Input: part model. Units: mm. Frame: model coordinates. Face numbers are marked on the shaded views. A direction names the side the tool comes from. Give positions to 0.01 mm unless a question says otherwise; leave off trailing zeros. Order: outer loops, then holes, each group sorted by start corner. A loop starts at its lowest first (then second) coordinate and runs counter-clockwise, first axis right, second up. Notation, with made-up numbers: (-6.75, -13) - (42.25, -13) arc R23 cw to (42.25, 3) - close; hole circle Ø10 at (8.25, 85.5). An arc over 180 degrees is marked (long way). Answer in a Markdown table with one row per item. Add a question column.
1. Section query B-B on y = 0.5. Return loops of the section in (x, z).
2. Mould query, pull axis Y, two halves, no side actions, for the marked faces 4, 5, 6 and 7. Classes: released by +Y, released by -Y, zero draft, split by the parting line, or undercut.
3. Contact query for flat-ended pins moving along their axis: pin 1 (2 mm diameter, centred on x = -11, z = -3.5, fed in from +Y); pin 2 (2.5 mm diameter, centred on y = 0, z = -3, fed in from +X); pin 3 (5 mm diameter, centred on y = -14.5, z = -5, fed in from -X). Output: stop coordinate, or through.
4. Section query C-C on x = -28. Return loops of the section in (y, z), and give its area (3 significant figures).
5. Access query for the marked faces 1, 2 and 3. Directions: +Z, -Z, +X, -X, +Y, -Y. A direction counts if a zero-diameter tool reaches every point of the face in a straight line with its end or side. Return the directions, or none.
6. Ray query, line 1 (Y direction, x = -19.5, z = -7.5); line 2 (X direction, y = -16.25, z = -1.75); line 3 (X direction, y = -7, z = -2.75). Return the intervals inside material, ascending. Write a range as [from, to].
Autodesk Inventor part; units mm, degrees
ref_plane "Work Plane2" through (-20.3233, -0.3, -20.2296) normal (0, 1, 0) x (0, 0, 1)
ref_plane "YZ Plane" through (0, 0, 0) normal (1, 0, 0) x (0, 1, 0)
ref_plane "XZ Plane" through (0, 0, 0) normal (0, 1, 0) x (-1, 0, 0)
sketch "Sketch1" plane through (0, 0, 0) normal (0, 0, 1) x (1, 0, 0)
  arc A0 (-31.9035, -17) -> (-29.9035, -19) centre (-29.9035, -17) ccw
  line L0 (-29.9035, -19) -> (-2, -19)
  arc A1 (-2, -19) -> (0, -17) centre (-2, -17) ccw
  line L1 (0, 1) -> (0, -17)
  arc A2 (0, 1) -> (-2, 3) centre (-2, 1) ccw
  line L2 (-2, 3) -> (-29.9035, 3)
  arc A3 (-29.9035, 3) -> (-31.9035, 1) centre (-29.9035, 1) ccw
  line L3 (-31.9035, -17) -> (-31.9035, 1)
  line L4 (-17.2029, -18.3) -> (-17.2029, -16)
  line L5 (-28.9035, -16) -> (-17.2029, -16)
  line L6 (-28.9035, 0) -> (-28.9035, -16)
  line L7 (-17.2029, 0) -> (-28.9035, 0)
  line L8 (-17.2029, 0) -> (-17.2029, 2.3)
  line L9 (-17.2029, 2.3) -> (-14.6938, 2.3)
  line L10 (-14.6938, 2.3) -> (-14.6938, 0)
  line L11 (-3, 0) -> (-14.6938, 0)
  line L12 (-3, 0) -> (-3, -16)
  line L13 (-14.6938, -16) -> (-3, -16)
  line L14 (-14.6938, -16) -> (-14.6938, -18.3)
  line L15 (-17.2029, -18.3) -> (-14.6938, -18.3)
  line L16 (-14.6938, -16) -> (-17.2029, -16)
  line L17 (-14.6938, 0) -> (-17.2029, 0)
  line L18 (-16.9029, -16) -> (-14.9938, -16)
  line L19 (-14.9938, -16) -> (-14.9938, -18)
  line L20 (-14.9938, -18) -> (-16.9029, -18)
  line L21 (-16.9029, -18) -> (-16.9029, -16)
  line L22 (-16.9029, 2) -> (-14.9938, 2)
  line L23 (-14.9938, 2) -> (-14.9938, 0)
  line L24 (-14.9938, 0) -> (-16.9029, 0)
  line L25 (-16.9029, 0) -> (-16.9029, 2)
  point P0 (0, 0)
  dimension "d5" = 0.3
  dimension "d6" = 0
  dimension "d7" = 0.3
  dimension "d8" = 0.3
  dimension "d9" = 0.3
  dimension "d10" = 0.3
  dimension "d11" = 0.3
  dimension "d12" = 0
extrude "Extrusion1" add sketch "Sketch1" against normal blind 14.9 contours L16 L19 L20 L21 | L25 L22 L23 L17
ref_plane "Work Plane1" through (0, 0, 0) normal (0, 0, 1) x (1, 0, 0)
sketch "Sketch2" plane through (0, 0, 0) normal (0, 0, 1) x (1, 0, 0)
  arc A0 (-31.9035, -17) -> (-29.9035, -19) centre (-29.9035, -17) ccw
  line L0 (-29.9035, -19) -> (-2, -19)
  arc A1 (-2, -19) -> (0, -17) centre (-2, -17) ccw
  line L1 (0, 1) -> (0, -17)
  arc A2 (0, 1) -> (-2, 3) centre (-2, 1) ccw
  line L2 (-2, 3) -> (-29.9035, 3)
  arc A3 (-29.9035, 3) -> (-31.9035, 1) centre (-29.9035, 1) ccw
  line L3 (-31.9035, -17) -> (-31.9035, 1)
  line L4 (-17.2029, -18.3) -> (-17.2029, -16)
  line L5 (-28.9035, -16) -> (-17.2029, -16)
  line L6 (-28.9035, 0) -> (-28.9035, -16)
  line L7 (-17.2029, 0) -> (-28.9035, 0)
  line L8 (-17.2029, 0) -> (-17.2029, 2.3)
  line L9 (-17.2029, 2.3) -> (-14.6938, 2.3)
  line L10 (-14.6938, 2.3) -> (-14.6938, 0)
  line L11 (-3, 0) -> (-14.6938, 0)
  line L12 (-3, 0) -> (-3, -16)
  line L13 (-14.6938, -16) -> (-3, -16)
  line L14 (-14.6938, -16) -> (-14.6938, -18.3)
  line L15 (-17.2029, -18.3) -> (-14.6938, -18.3)
  line L16 (-17.2029, 0) -> (-14.6938, 0)
  line L17 (-14.6938, 0) -> (-14.6938, 2.3)
  line L18 (-14.6938, 2.3) -> (-17.2029, 2.3)
  line L19 (-17.2029, 2.3) -> (-17.2029, 0)
  line L20 (-17.2029, -18.3) -> (-14.6938, -18.3)
  line L21 (-14.6938, -18.3) -> (-14.6938, -16)
  line L22 (-14.6938, -16) -> (-17.2029, -16)
  line L23 (-17.2029, -16) -> (-17.2029, -18.3)
  point P0 (0, 0)
extrude "Extrusion2" add sketch "Sketch2" along normal blind 3 contours L3 A3 L2 A2 L1 A1 L0 A0 | L4 L22 L14 L15 | L5 L6 L7 L16 L11 L12 L13 L22 | L8 L9 L10 L16
fillet "Fillet1" radius 2 8 edges at (-31.3177, -18.4142, 3) (-31.9035, -8, 3) (-31.3177, 2.4142, 3) (-15.9518, 3, 3) (-0.5858, 2.4142, 3) (0, -8, 3) (-0.5858, -18.4142, 3) (-15.9518, -19, 3)
sketch "Sketch3" plane through (0, 0, 0) normal (0, 0, -1) x (-1, 0, 0)
  arc A0 (29.9035, -19) -> (31.9035, -17) centre (29.9035, -17) ccw
  line L0 (29.9035, -19) -> (2, -19)
  arc A1 (0, -17) -> (2, -19) centre (2, -17) ccw
  line L1 (0, 1) -> (0, -17)
  arc A2 (2, 3) -> (0, 1) centre (2, 1) ccw
  line L2 (2, 3) -> (29.9035, 3)
  arc A3 (31.9035, 1) -> (29.9035, 3) centre (29.9035, 1) ccw
  line L3 (31.9035, -17) -> (31.9035, 1)
  line L4 (17.2029, -18.3) -> (17.2029, -16)
  line L5 (28.9035, -16) -> (17.2029, -16)
  line L6 (28.9035, 0) -> (28.9035, -16)
  line L7 (17.2029, 0) -> (28.9035, 0)
  line L8 (17.2029, 0) -> (17.2029, 2.3)
  line L9 (17.2029, 2.3) -> (14.6938, 2.3)
  line L10 (14.6938, 2.3) -> (14.6938, 0)
  line L11 (3, 0) -> (14.6938, 0)
  line L12 (3, 0) -> (3, -16)
  line L13 (14.6938, -16) -> (3, -16)
  line L14 (14.6938, -16) -> (14.6938, -18.3)
  line L15 (17.2029, -18.3) -> (14.6938, -18.3)
  line L16 (14.9938, 0) -> (16.9029, 0)
  line L17 (14.9938, 0) -> (14.9938, -0.3)
  line L18 (14.9938, -0.3) -> (3.3, -0.3)
  line L19 (3.3, -0.3) -> (3.3, -1.8)
  line L20 (3.3, -1.8) -> (28.6035, -1.8)
  line L21 (28.6035, -0.3) -> (16.9029, -0.3)
  line L22 (16.9029, 0) -> (16.9029, -0.3)
  line L23 (28.6035, -1.8) -> (28.6035, -0.3)
  line L24 (3, -8) -> (28.9035, -8) construction
  line L25 (14.9938, -16) -> (16.9029, -16)
  line L26 (14.9938, -16) -> (14.9938, -15.7)
  line L27 (14.9938, -15.7) -> (3.3, -15.7)
  line L28 (3.3, -15.7) -> (3.3, -14.2)
  line L29 (3.3, -14.2) -> (28.6035, -14.2)
  line L30 (28.6035, -15.7) -> (16.9029, -15.7)
  line L31 (16.9029, -16) -> (16.9029, -15.7)
  line L32 (28.6035, -14.2) -> (28.6035, -15.7)
  line L33 (3.3, -1.8) -> (3.3, -14.2)
  line L34 (4.8, -14.2) -> (4.8, -1.8)
  line L35 (28.6035, -1.8) -> (28.6035, -14.2)
  line L36 (27.1035, -14.2) -> (27.1035, -1.8)
  point P0 (0, 0)
  dimension "d13" = 0.3
  dimension "d14" = 0.3
  dimension "d15" = 1.5
  dimension "d16" = 0.3
  dimension "d17" = 0.3
  dimension "d20" = 1.5
  dimension "d21" = 1.5
extrude "Extrusion3" add sketch "Sketch3" along normal blind 3 contours L16 L22 L21 L23 L20 L19 L18 L17 | L20 L34 L29 L33 | L35 L29 L36 L20 | L29 L32 L30 L31 L25 L26 L27 L28
sketch "Sketch4" plane through (-14.9938, -18, -14.9) normal (1, 0, 0) x (0, 0, -1)
  line L0 (-14.9, -0.3) -> (2.2893, -0.3)
  line L1 (-14.9, 2) -> (-14.9, -0.3)
  line L2 (2.2893, 2) -> (-14.9, 2)
  line L3 (2.2893, 2) -> (2.2893, -0.3)
  line L4 (0, 2) -> (0, 0)
  line L5 (-14.9, 0) -> (0, 0)
  line L6 (-14.9, 2.3) -> (-14.9, 0)
  line L7 (-14.9, 2.3) -> (-11.9, 2.3)
  line L8 (-11.9, 2.3) -> (-11.9, 2)
  line L9 (-11.9, 2) -> (0, 2)
  line L10 (0, 18) -> (0, 20)
  line L11 (-14.9, 20) -> (0, 20)
  line L12 (-14.9, 20) -> (-14.9, 17.7)
  line L13 (-14.9, 17.7) -> (-11.9, 17.7)
  line L14 (-11.9, 17.7) -> (-11.9, 18)
  line L15 (-11.9, 18) -> (0, 18)
  line L16 (-7.45, 2) -> (-11.9, 4.6913)
  line L17 (-11.9, 4.6913) -> (-11.9, 2.3)
  line L18 (-11.9, 10) -> (3.9744, 10) construction
  line L19 (-7.45, 18) -> (-11.9, 15.3087)
  line L20 (-11.9, 15.3087) -> (-11.9, 17.7)
  point P0 (-14.9, 18)
extrude "Extrusion4" add sketch "Sketch4" against normal up to surface (1.9092 mm away) contours L8 L17 L16 L2 | L19 L20 L14 L15
sketch "Sketch6" plane through (0, 0, 0) normal (0, 0, -1) x (-1, 0, 0)
  line L0 (27.1035, -1.8) -> (4.8, -1.8)
  line L1 (4.8, -1.8) -> (4.8, -14.2)
  line L2 (4.8, -14.2) -> (27.1035, -14.2)
  line L3 (27.1035, -14.2) -> (27.1035, -1.8)
  line L4 (14.9938, -13.3087) -> (16.9029, -13.3087)
  line L5 (14.9938, -2.6913) -> (16.9029, -2.6913)
  line L6 (14.9938, -2.6913) -> (5.6913, -2.6913)
  line L7 (5.6913, -2.6913) -> (5.6913, -13.3087)
  line L8 (5.6913, -13.3087) -> (14.9938, -13.3087)
  line L9 (16.9029, -13.3087) -> (26.2122, -13.3087)
  line L10 (26.2122, -13.3087) -> (26.2122, -2.6913)
  line L11 (26.2122, -2.6913) -> (16.9029, -2.6913)
  point P0 (0, 0)
  dimension "d24" = 0.8913
  dimension "d25" = 0.8913
  dimension "d26" = 0.8913
extrude "Extrusion5" add sketch "Sketch6" along normal up to surface (3 mm away)
sketch "Sketch7" plane through (0, 0, 0) normal (0, 0, -1) x (-1, 0, 0)
  line L0 (14.9938, -2.6913) -> (14.9938, -0.3)
  line L1 (3.3, -0.3) -> (14.9938, -0.3)
  line L2 (3.3, -15.7) -> (3.3, -0.3)
  line L3 (14.9938, -15.7) -> (3.3, -15.7)
  line L4 (14.9938, -13.3087) -> (14.9938, -15.7)
  line L5 (5.6913, -13.3087) -> (14.9938, -13.3087)
  line L6 (5.6913, -2.6913) -> (5.6913, -13.3087)
  line L7 (14.9938, -2.6913) -> (5.6913, -2.6913)
  line L8 (16.9029, -0.3) -> (16.9029, -2.6913)
  line L9 (26.2122, -2.6913) -> (16.9029, -2.6913)
  line L10 (26.2122, -13.3087) -> (26.2122, -2.6913)
  line L11 (16.9029, -13.3087) -> (26.2122, -13.3087)
  line L12 (16.9029, -13.3087) -> (16.9029, -15.7)
  line L13 (28.6035, -15.7) -> (16.9029, -15.7)
  line L14 (28.6035, -0.3) -> (28.6035, -15.7)
  line L15 (16.9029, -0.3) -> (28.6035, -0.3)
  line L16 (5.6913, -8) -> (10.3425, -13.3087)
  line L17 (5.6913, -8) -> (10.3425, -2.6913)
  line L18 (21.5576, -2.6913) -> (26.2122, -8)
  line L19 (26.2122, -8) -> (21.5576, -13.3087)
  point P0 (0, 0)
extrude "Extrusion6" add sketch "Sketch7" along normal up to surface (3 mm away) contours L17 L6 L7 | L16 L5 L6 | L9 L10 L18 | L10 L11 L19
sketch "Sketch8" plane through (0, 0, -14.9) normal (0, 0, -1) x (-1, 0, 0)
  line L0 (16.9029, 2) -> (16.9029, 0)
  line L1 (14.9938, 0) -> (14.9938, 2)
  line L2 (16.9029, 0) -> (14.9938, 0)
  line L3 (13.4938, 2) -> (18.4028, 2)
  line L4 (18.4028, 2) -> (18.4028, 0)
  line L5 (18.4028, 0) -> (13.4938, 0)
  line L6 (13.4938, 0) -> (13.4938, 2)
  line L7 (3.3, -15.7) -> (3.3, -0.3)
  line L8 (28.6035, -0.3) -> (28.6035, -15.7)
  line L9 (3.3, -8) -> (28.6035, -8) construction
  line L10 (13.4938, -18) -> (18.4028, -18)
  line L11 (18.4028, -18) -> (18.4028, -16)
  line L12 (18.4028, -16) -> (13.4938, -16)
  line L13 (13.4938, -16) -> (13.4938, -18)
  point P0 (0, 0)
  dimension "d31" = 4.909
  dimension "d32" = 1.9092
  dimension "d33" = 1.4999
  dimension "d34" = 0
  dimension "d35" = 2
  dimension "d36" = 2
extrude "Extrusion7" add sketch "Sketch8" against normal up to surface (14.9 mm away)
sketch "Sketch9" plane through (-14.9938, -16, 0) normal (1, 0, 0) x (0, 0, -1)
  line L0 (0, 0) -> (7.45, 0)
  line L1 (7.45, 0) -> (3, 2.6913)
  line L2 (3, 2.6913) -> (3, 0.3)
  line L3 (0, 0.3) -> (3, 0.3)
  line L4 (0, 0) -> (0, 0.3)
  line L5 (7.45, 16) -> (0, 16)
  line L6 (0, 16) -> (0, 15.7)
  line L7 (0, 15.7) -> (3, 15.7)
  line L8 (3, 13.3087) -> (3, 15.7)
  line L9 (3, 13.3087) -> (7.45, 16)
  point P0 (0, 16)
extrude "Extrusion8" add sketch "Sketch9" along normal up to surface (1.4999 mm away)
sketch "Sketch10" plane through (-16.9029, -16, 0) normal (-1, 0, 0) x (0, 0, 1)
  line L0 (-7.45, 0) -> (0, 0)
  line L1 (0, 0.3) -> (0, 0)
  line L2 (0, 0.3) -> (-3, 0.3)
  line L3 (-3, 2.6913) -> (-3, 0.3)
  line L4 (-7.45, 0) -> (-3, 2.6913)
  line L5 (0, 16) -> (-7.45, 16)
  line L6 (-3, 13.3087) -> (-7.45, 16)
  line L7 (-3, 15.7) -> (-3, 13.3087)
  line L8 (0, 15.7) -> (-3, 15.7)
  line L9 (0, 16) -> (0, 15.7)
  point P0 (0, 16)
extrude "Extrusion9" add sketch "Sketch10" along normal up to surface (1.4999 mm away)
sketch "Sketch11" plane through (-21.5576, -2.6913, 0) normal (0, -1, 0) x (1, 0, 0)
  line L0 (11.2151, -3) -> (11.2151, 0)
  line L1 (0, 0) -> (11.2151, 0)
  line L2 (0, 0) -> (0, -3)
  line L3 (0, -3) -> (3.1547, -3)
  line L4 (3.1547, -3) -> (8.0637, -3)
  line L5 (8.0637, -3) -> (11.2151, -3)
  line L6 (8.0637, -7.45) -> (3.1547, -7.45)
  line L7 (3.1547, -3) -> (3.1547, -7.45)
  line L8 (8.0637, -7.45) -> (8.0637, -3)
  point P0 (21.5576, 0)
extrude "Extrusion10" cut sketch "Sketch11" against normal blind 0.4
sketch "Sketch12" plane through (-21.5576, -13.3087, 0) normal (0, 1, 0) x (1, 0, 0)
  line L0 (11.2151, 0) -> (11.2151, 3)
  line L1 (11.2151, 3) -> (8.0637, 3)
  line L2 (8.0637, 3) -> (3.1547, 3)
  line L3 (3.1547, 3) -> (0, 3)
  line L4 (0, 3) -> (0, 0)
  line L5 (11.2151, 0) -> (0, 0)
  line L6 (8.0637, 3.6614) -> (3.1547, 3.6614)
  line L7 (3.1547, 3.6614) -> (3.1547, 3)
  line L8 (8.0637, 3.6614) -> (8.0637, 3)
  point P0 (21.5576, 0)
extrude "Extrusion11" cut sketch "Sketch12" against normal blind 0.4
sketch "Sketch13" plane through (-18.4028, 0, -7.45) normal (0, -1, 0) x (1, 0, 0)
  line L0 (4.909, 0) -> (0, 0)
  line L1 (0, -7.45) -> (0, 0)
  line L2 (0, -7.45) -> (4.909, -7.45)
  line L3 (4.909, -7.45) -> (4.909, 0)
  point P0 (18.4028, 7.45)
ref_plane "Work Plane2" through (-20.3233, -0.3, -20.2296) normal (0, 1, 0) x (0, 0, 1)
extrude "Extrusion12" add sketch "Sketch13" along normal up to surface (0.3 mm away)
sketch "Sketch14" plane through (-18.4028, 2, -14.9) normal (0, 1, 0) x (1, 0, 0)
  line L0 (4.909, 0) -> (0, 0)
  line L1 (0, 0) -> (0, -14.9)
  line L2 (6.8295, -3.4204) -> (-1.9205, -3.4204)
  line L3 (0, -3.4204) -> (4.909, -3.4204)
  line L4 (4.909, -3.4204) -> (4.909, 0)
  line L5 (4.909, 0) -> (0, 0)
  line L6 (0, 0) -> (0, -3.4204)
  point P0 (18.4028, -14.9)
extrude "Extrusion13" cut sketch "Sketch14" against normal up to surface (20 mm away)
ref_plane "Work Plane3" through (-20.3233, -0.3, -11.4796) normal (0, 0, 1) x (-1, 0, 0)
sketch "Sketch15" plane through (-20.3233, -0.3, -11.4796) normal (0, 0, 1) x (-1, 0, 0)
  line L0 (-8.75, 17.6961) -> (-8.75, 13)
  line L1 (0, 17.6961) -> (-8.75, 17.6961)
  line L2 (-8.75, 13) -> (0, 13)
  line L3 (0, 17.6961) -> (0, 13)
  line L4 (-8.75, 2.4) -> (-8.75, -2.3)
  line L5 (0, 2.4) -> (-8.75, 2.4)
  line L6 (-8.75, -2.3) -> (0, -2.3)
  line L7 (0, -2.3) -> (0, 2.4)
  point P0 (-20.3233, -0.3)
extrude "Extrusion14" add sketch "Sketch15" along normal up to surface (11.4796 mm away)
equation "\"d7\" = d5"
equation "\"d8\" = d5"
equation "\"d9\" = d5"
equation "\"d10\" = d9"
equation "\"d11\" = d10"
equation "\"d20\" = d15"
equation "\"d21\" = d20"
equation "\"d25\" = d24"
equation "\"d26\" = d24"
equation "\"d33\" = -0.5 * d32 + 0.5 * d31"
equation "\"d35\" = d36"
properties part number "GearBoxTop"
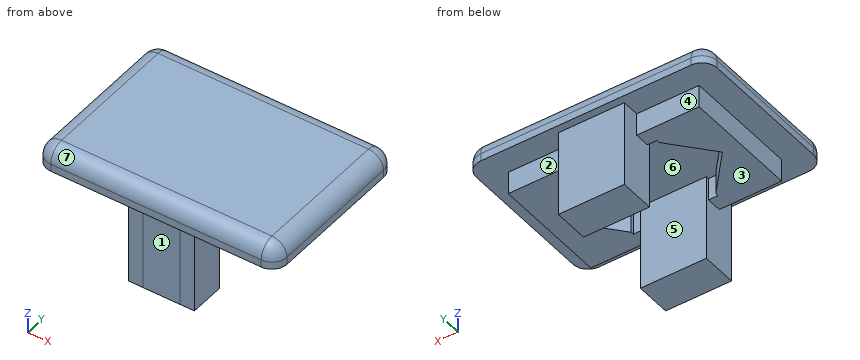
Answer:
| question | item | result |
|---|---|---|
| 1 | outline | (-31.9, 0) - (-20.32, 0) - (-20.32, -11.48) - (-11.57, -11.48) - (-11.57, 0) - (0, 0) - (0, 1) arc R2 ccw to (-2, 3) - (-29.9, 3) arc R2 ccw to (-31.9, 1) - close |
| 2 | face 4 | released by +Y |
| 2 | face 5 | undercut |
| 2 | face 6 | undercut |
| 2 | face 7 | released by -Y |
| 3 | pin 1 | stops at y = 2 |
| 3 | pin 2 | stops at x = -3.3 |
| 3 | pin 3 | stops at x = -28.6 |
| 4 | outline | (-19, 0) - (-15.7, 0) - (-15.7, -3) - (-0.3, -3) - (-0.3, 0) - (3, 0) - (3, 1) arc R2 ccw to (1, 3) - (-17, 3) arc R2 ccw to (-19, 1) - close |
| 4 | area | 110 mm² |
| 5 | face 1 | -Z, +X, -X, -Y |
| 5 | face 2 | -Z, +X, +Y |
| 5 | face 3 | -Z, -X, +Y, -Y |
| 6 | line 1 | y = [-18, -13.3], [-2.7, 2] |
| 6 | line 2 | x = [-20.32, -11.57] |
| 6 | line 3 | x = [-28.6, -25.34], [-6.57, -3.3] |
